```python
from build123d import *

# Parameters (mm, degrees)
CROQUIS1_W              = 150
CROQUIS1_H              = 150
SALIENTE_EXTRUIR1_DEPTH = 2
CROQUIS2_R              = 2
CROQUIS2_R_2            = 7
CROQUIS2_R_3            = 1.5
CROQUIS2_W              = 5
CROQUIS2_H              = 15
CORTAR_EXTRUIR1_DEPTH   = 2


with BuildPart() as part:
    # Croquis1 → Saliente-Extruir1 (new body)
    with BuildSketch(Plane.XY):
        Rectangle(CROQUIS1_W, CROQUIS1_H)
    extrude(amount=SALIENTE_EXTRUIR1_DEPTH)

    # Croquis2 → Cortar-Extruir1 (cut)
    with BuildSketch(Plane.XY.offset(2)):
        with Locations((-67.5, -67.5)):
            Circle(CROQUIS2_R)
        with Locations((67.5, -67.5)):
            Circle(CROQUIS2_R)
        with Locations((67.5, 67.5)):
            Circle(CROQUIS2_R)
        with Locations((-67.5, 67.5)):
            Circle(CROQUIS2_R)
        Circle(CROQUIS2_R_2)
        with Locations((-15, -15)):
            Circle(CROQUIS2_R)
        with Locations((15, -15)):
            Circle(CROQUIS2_R)
        with Locations((15, 15)):
            Circle(CROQUIS2_R)
        with Locations((-15, 15)):
            Circle(CROQUIS2_R)
        with Locations((-10.52379439, 25.406687144)):
            Circle(CROQUIS2_R_3)
        with Locations((10.52379439, 25.406687144)):
            Circle(CROQUIS2_R_3)
        with Locations((25.406687144, 10.52379439)):
            Circle(CROQUIS2_R_3)
        with Locations((25.406687144, -10.52379439)):
            Circle(CROQUIS2_R_3)
        with Locations((10.52379439, -25.406687144)):
            Circle(CROQUIS2_R_3)
        with Locations((-10.52379439, -25.406687144)):
            Circle(CROQUIS2_R_3)
        with Locations((-27.5, 0)):
            Rectangle(CROQUIS2_W, CROQUIS2_H)
    extrude(amount=-CORTAR_EXTRUIR1_DEPTH, mode=Mode.SUBTRACT)


solid = part.part
```
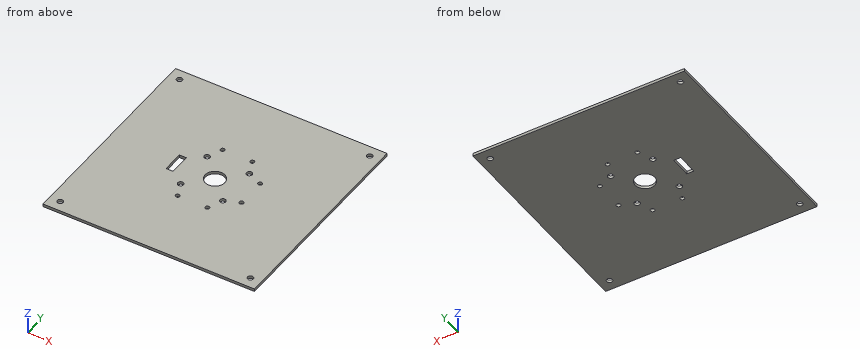
Geometry: final body of the model. Coordinates: model frame, mm. Round coordinates to 2 decimals unless told otherwise and drop trailing zeros. Order: outer loops, then holes, each group sorted by start corner. A loop starts at its lowest first (then second) coordinate and runs counter-clockwise, first axis right, second up. Notation, with made-up numbers: (10.5, 83.25) - (39.5, 83.25) arc R22 cw to (39.5, 100.25) - close; hole circle Ø7 at (-38, 33). An arc over 180 degrees is marked (long way). Use CSV: the item, a comma, the result in double quotes. Start each with the question number.
Q1. Section query C-C (z = 1.45). State how many separate pieces and enclosed holes the cut face has, and give its area (3 significant figures).
Q2. First-contact query: pin 1 (3.5 mm diameter, centred on x = -67.5, y = -67.5, fed in from +Z). Flat tip, straight axial feed; report the tip coordinate or a pass-through.
Q3. Section query A-A (y = 67.5). Return loops of the section in (x, z), and give its area (3 significant figures).
Q4. Material intervals for line 1 along Y through (x, z) = (-10.5, 1.5); line 2 along Y through (x, z) = (-67.5, 0.8); line 3 along X through (y, z) = (-67, 0.3), sorted ascending. Write a range as from..to.
Result set:
1,separate pieces,"1"
1,enclosed holes,"16"
1,area,"22,100 mm2"
2,pin 1,"passes through"
3,outline,"(-75, 0) - (-69.5, 0) - (-69.5, 2) - (-75, 2) - close; (-65.5, 0) - (65.5, 0) - (65.5, 2) - (-65.5, 2) - close; (69.5, 0) - (75, 0) - (75, 2) - (69.5, 2) - close"
3,area,"284 mm2"
4,line 1,"y = -75..-26.91, -23.91..23.91, 26.91..75"
4,line 2,"y = -75..-69.5, -65.5..65.5, 69.5..75"
4,line 3,"x = -75..-69.44, -65.56..65.56, 69.44..75"
